Read the model definition and answer for the solid it produces. Units are mm, in the model's axes. A direction names the side the tool comes from. Coordinates: 2 decimals unless noted, no trailing zeros. Write each loop counter-clockwise with the first axis right and the second up, starting at its lowest first coordinate (ties: lowest second). Pieces come first, ordered by that corner, then holes.
(1) The mould has two halves that part along Z. Classify faces 1 (the flat face through (-71.267, -64, -102)), 2 (the flat face through (-68.727, -64, -104)), 3 (the flat face through (19, -64, 24.629)): +Z half, -Z half, draft (parallel to the pull), parting line (faces both ways), or undercut.
(2) Find the intervals of material crossed by probe 1 along Y at (x, z) = (-102.5, 135); probe 2 along Z at (x, y) = (41.5, -80); probe 3 along Z at (x, y) = (-119.5, -52), in increasing order.
(3) Section C-C on z = 139.5 is taken. Write down the section's boundary in (x, y).
(4) Section B-B on y = -114.5 is taken. Write down the section's boundary in (x, z), then the cut area to 3 significant figures.
(5) Section D-D on x = -140 is taken. Write down the section's boundary in (y, z).
(6) Which of the six approach directions +Z, -Z, +X, -X, +Y, -Y give full straight-line access (tool end or side, diameter ignored) to faces 4 (the flat face through (-80, -2.54, 53)), 5 (the flat face through (-45, -63, 227.829))?
(7) Section A-A on x = 54 is taken. Write down the section's boundary in (y, z), then the cut area to 3 significant figures.
(8) Given pin 1 (1 mm diameter, centred on y = -19, z = -24.5, fed in from +X), flat-ended and moving along its own axis, determine where the tip first touches the part or whether it passes through.
from build123d import *

# Parameters (mm, degrees)
F0_W     = 304.8
F0_H     = 457.2
F1_DEPTH = 127
F2_W     = 177.8
F2_H     = 254
F3_DEPTH = 127
F4_T     = -2.54


with BuildPart() as f1:
    # F0 (on Front) → F1 (new body)
    with BuildSketch(Plane.XZ):
        with Locations((-43.326701003, -0.7706172764)):
            Rectangle(F0_W, F0_H)
    extrude(amount=F1_DEPTH)

    # F2 (on face) → F3 (cut)
    with BuildSketch(Plane.XZ.offset(127)):
        with Locations((20.173298997, -102.3706172764)):
            Rectangle(F2_W, F2_H)
    extrude(amount=-F3_DEPTH, mode=Mode.SUBTRACT)

    # F4
    f4_openings = [f1.faces().sort_by_distance(p)[0] for p in [
        (-195.726701, -63.5, -0.770617),
    ]]
    offset(amount=F4_T, openings=f4_openings, kind=Kind.INTERSECTION)


solid = f1.part
Response:
1. face 1: undercut
1. face 2: draft
1. face 3: -Z half
2. probe 1: y = -127 to -124.46, -2.54 to 0
2. probe 2: z = 24.63 to 27.17, 225.29 to 227.83
2. probe 3: z = -229.37 to -226.83, 225.29 to 227.83
3. outline: (-195.73, -127) - (109.07, -127) - (109.07, 0) - (-195.73, 0) - (-195.73, -2.54) - (106.53, -2.54) - (106.53, -124.46) - (-195.73, -124.46) - close
4. outline: (-195.73, -229.37) - (-68.73, -229.37) - (-68.73, 24.63) - (109.07, 24.63) - (109.07, 227.83) - (-195.73, 227.83) - (-195.73, 225.29) - (106.53, 225.29) - (106.53, 27.17) - (-71.27, 27.17) - (-71.27, -226.83) - (-195.73, -226.83) - close
4. area: 2,700 mm2
5. outline: (-127, -229.37) - (0, -229.37) - (0, 227.83) - (-127, 227.83) - close; hole (-124.46, -226.83) - (-2.54, -226.83) - (-2.54, 225.29) - (-124.46, 225.29) - close
6. face 4: -X
6. face 5: +Z, +X, -X, +Y, -Y
7. outline: (-127, 24.63) - (0, 24.63) - (0, 227.83) - (-127, 227.83) - close; hole (-124.46, 27.17) - (-2.54, 27.17) - (-2.54, 225.29) - (-124.46, 225.29) - close
7. area: 1,650 mm2
8. pin 1: stops at x = -68.73
